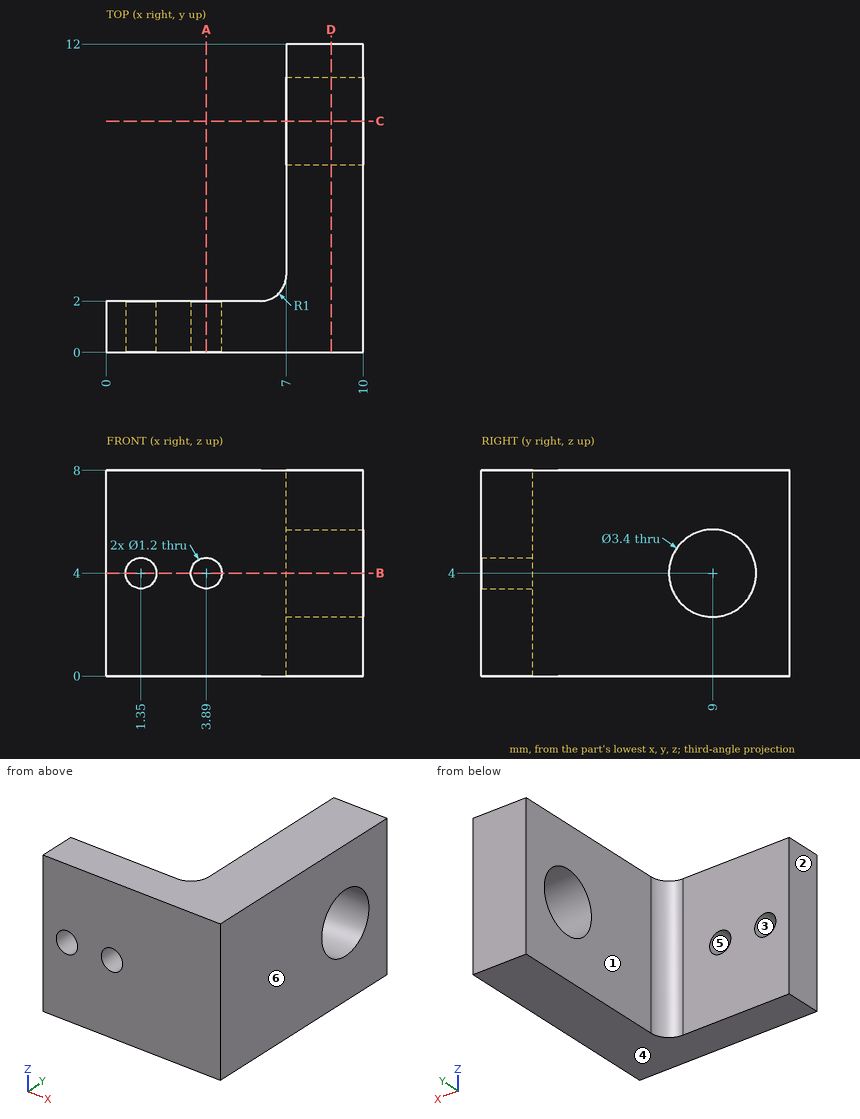
Source: three-view drawing plus pictorial views. Frame: mm from the lowest corner of the part. A direction names the side the tool comes from. Give positions to 0.01 mm unless a question says otherwise; leave off trailing zeros. Order: outer loops, then holes, each group sorted by start corner. A loop starts at its lowest first (then second) coordinate and runs counter-clockwise, first axis right, second up. Notation, with made-up numbers: M -21,61.25 L 4,61.25 A31 ccw 4,87.25 Z; hole C 55.5,36 d2. An arc over 180 degrees is marked long. One line per question, with ' | ' between items.
1) Contact query for flat-ended pins moving along their axis: P1, Ø1.6, axis at x = 1.35, z = 4, coming from the -Y side; P2, Ø3, axis at y = 9, z = 4, coming from the -X side; P3, Ø3, axis at y = 4, z = 4, coming from the -X side. Output: stop coordinate, or through.
Filled in:
P1: stops at y = 0 | P2: passes through | P3: stops at x = 6.87
2) Access query for the marked faces 1 and 2. Directions: +Z, -Z, +X, -X, +Y, -Y. A direction counts if a zero-diameter tool reaches every point of the face in a straight line with its end or side. Return the directions, or none.
Filled in:
face 1: +Z, -Z, -X, +Y | face 2: +Z, -Z, -X, +Y, -Y
3) Section A-A on x = 3.89. Output: boundary loops of the cut face in (y, z).
Filled in:
outline: M 0,0 L 2,0 L 2,3.4 L 0,3.4 Z; M 0,4.6 L 2,4.6 L 2,8 L 0,8 Z
4) Draft query along Z for the marked faces 3, 4, 5 and 6. Return one class per face: pulls with the +Z half, pulls with the -Z half, needs draft (parallel to the pull), parting line crosses it, or undercut.
Filled in:
face 3: undercut | face 4: pulls with the -Z half | face 5: undercut | face 6: needs draft
5) Ray query, L1, parallel to Y at x = 9.05, z = 4; L2, parallel to X at y = 8.25, z = 1.75; L3, parallel to Y at x = 5.25, z = 1. Return the intervals inside material, ascending.
Filled in:
L1: y = 0 to 7.3, 10.7 to 12 | L2: x = 7 to 10 | L3: y = 0 to 2
6) Section B-B on z = 4. Output: boundary loops of the cut face in (x, y).
Filled in:
outline: M 0,0 L 0.75,0 L 0.75,2 L 0,2 Z; M 1.95,0 L 3.29,0 L 3.29,2 L 1.95,2 Z; M 4.49,0 L 10,0 L 10,7.3 L 7,7.3 L 7,3 A1 cw 6,2 L 4.49,2 Z; M 7,10.7 L 10,10.7 L 10,12 L 7,12 Z
7) Section C-C on y = 9. Output: boundary loops of the cut face in (x, z), and give its area (3 significant figures).
Filled in:
outline: M 7,0 L 10,0 L 10,2.3 L 7,2.3 Z; M 7,5.7 L 10,5.7 L 10,8 L 7,8 Z | area: 13.8 mm2
8) Section D-D on x = 8.75. Output: boundary loops of the cut face in (y, z), and give its area (3 significant figures).
Filled in:
outline: M 0,0 L 12,0 L 12,8 L 0,8 Z; hole C 9,4 d3.4 | area: 86.9 mm2
